The model under review builds one solid part; all positions refer to its coordinate system, in mm. Coordinates: 2 decimals unless noted, no trailing zeros. Write each loop counter-clockwise with the first axis right and the second up, starting at its lowest first coordinate (ties: lowest second). Pieces come first, ordered by that corner, then holes.
1) Add section C-C, the plane x = 86.5. State the section outline as (y, z) points (3 decimals).
2) For line 1 (Z direction, x = 34, y = 0.3); line 2 (X direction, y = 2.85, z = -106.5); line 3 (X direction, y = 2.9, z = 31.5), list the stretches that pass through material, from the lowest coordinate up.
3) Add section B-B, the plane z = -87.5. State the section outline as (x, y) points (3 decimals), then the cut area to 3 significant figures.
4) Add section D-D, the plane z = 97. State the section outline as (x, y) points (3 decimals), then the cut area to 3 significant figures.
5) Add section A-A, the plane y = 2.05. Give the number of separate pieces and of enclosed holes in the cut face, then the cut area to 3 significant figures.
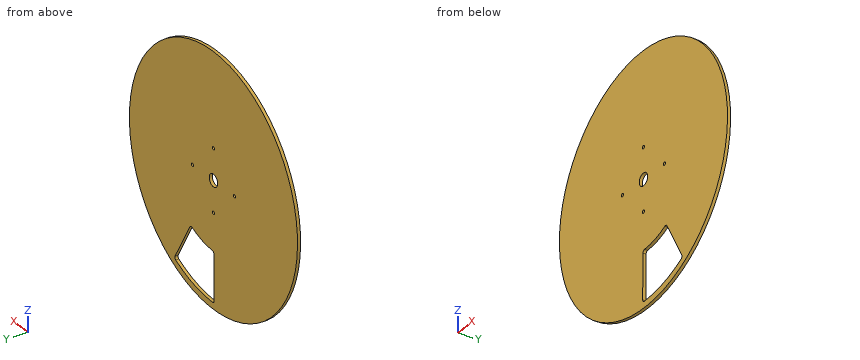
from build123d import *

# Parameters (mm, degrees)
SKETCH1_R           = 127
BOSS_EXTRUDE1_DEPTH = 3.175
SKETCH2_R           = 6.35
CUT_EXTRUDE1_DEPTH  = 180.63318353
CUT_EXTRUDE2_DEPTH  = 180.63318353
SKETCH4_R           = 1.5875
CUT_EXTRUDE3_DEPTH  = 180.63318353
CIRPATTERN1_COUNT   = 4
FILLET1_R           = 2.54


with BuildPart() as part:
    # Sketch1 → Boss-Extrude1 (new body)
    with BuildSketch(Plane(origin=(0, 0, 0), x_dir=(1, 0, 0), z_dir=(0, 1, 0))):
        with Locations(Location((0, 0, 0), (0, 0, 270))):
            Circle(SKETCH1_R)
    extrude(amount=BOSS_EXTRUDE1_DEPTH)

    # Sketch2 → Cut-Extrude1 (cut, through all)
    with BuildSketch(Plane(origin=(0, 3.175, 0), x_dir=(1, 0, 0), z_dir=(0, 1, 0))):
        with Locations(Location((0, 0, 0), (0, 0, 270))):
            Circle(SKETCH2_R)
    extrude(amount=-CUT_EXTRUDE1_DEPTH, mode=Mode.SUBTRACT)

    # Sketch3 → Cut-Extrude2 (cut, through all)
    with BuildSketch(Plane(origin=(0, 3.175, 0), x_dir=(1, 0, 0), z_dir=(0, 1, 0))):
        with BuildLine():
            Line((-0.69608151, 69.707591228), (-1.204718825, 120.643985149))
            ThreePointArc((-1.204718825, 120.643985149), (30.046443244, 116.817986877), (59.221085226, 104.981025331))
            Line((59.221085226, 104.981025331), (34.319233166, 60.837593106))
            ThreePointArc((34.319233166, 60.837593106), (17.387075213, 67.544440681), (-0.69608151, 69.707591228))
        make_face()
    extrude(amount=-CUT_EXTRUDE2_DEPTH, mode=Mode.SUBTRACT)

    # Sketch4 → Cut-Extrude3 (cut, through all)
    with BuildSketch(Plane(origin=(0, 3.175, 0), x_dir=(1, 0, 0), z_dir=(0, 1, 0))):
        with Locations(Location((0, -31.75, 0), (0, 0, 270))):
            Circle(SKETCH4_R)
    cut_extrude3 = extrude(amount=-CUT_EXTRUDE3_DEPTH, mode=Mode.SUBTRACT)

    # CirPattern1: Cut-Extrude3 ×4 about axis
    cirpattern1_axis = Axis((0, 0, 0), (0, 1, 0))
    for i in range(1, CIRPATTERN1_COUNT):
        add(cut_extrude3.rotate(cirpattern1_axis, i * 360 / CIRPATTERN1_COUNT), mode=Mode.SUBTRACT)

    # Fillet1
    fillet1_edges = [part.edges().sort_by_distance(p)[0] for p in [
        (34.319233166, 1.5875, -60.837593106),
        (-0.69608151, 1.5875, -69.707591228),
        (-1.204718825, 1.5875, -120.643985149),
        (59.221085226, 1.5875, -104.981025331),
    ]]
    fillet(fillet1_edges, radius=FILLET1_R)


solid = part.part
Geometry results:
1. outline: (0, -92.988) - (3.175, -92.988) - (3.175, 92.988) - (0, 92.988) - close
2. line 1: z = -122.36 to -115.72, -61.8 to 122.36
2. line 2: x = -69.19 to -1.06, 56.47 to 69.19
2. line 3: x = -123.03 to -1.57, 1.57 to 123.03
3. outline: (-92.048, 0) - (-0.874, 0) - (-0.874, 3.175) - (-92.048, 3.175) - close; (49.36, 0) - (92.048, 0) - (92.048, 3.175) - (49.36, 3.175) - close
3. area: 425 mm2
4. outline: (-81.976, 0) - (81.976, 0) - (81.976, 3.175) - (-81.976, 3.175) - close
4. area: 521 mm2
5. separate pieces: 1
5. enclosed holes: 6
5. area: 48,000 mm2
